```python
from build123d import *

# Parameters (mm, degrees)
SKETCH1_W           = 120.675
SKETCH1_H           = 1.5875
SKETCH6_R           = 7.9375
BOSS_EXTRUDE1_DEPTH = 101.6
SKETCH7_R           = 23.308025585
CUT_EXTRUDE3_DEPTH  = 19.075
SKETCH4_R           = 12.7
CUT_EXTRUDE4_DEPTH  = 41.50106


with BuildPart() as part:
    # Sketch1 → Revolve1 (revolve)
    with BuildSketch(Plane(origin=(0, 0, 0), x_dir=(1, 0, 0), z_dir=(0, 1, 0))):
        with Locations((79.5875, 8.73125)):
            Rectangle(SKETCH1_W, SKETCH1_H)
    revolve(axis=Axis((157.324, 0, 0), (-1, 0, 0)))

    # Sketch6 → Boss-Extrude1 (add)
    with BuildSketch(Plane.ZY.offset(-19.25)):
        with Locations(Location((0, 0, 0), (0, 0, 180))):
            Circle(SKETCH6_R)
    extrude(amount=-BOSS_EXTRUDE1_DEPTH)

    # Sketch7 → Cut-Extrude3 (cut)
    with BuildSketch(Plane(origin=(120.85, 0, 0), x_dir=(0, 0, -1), z_dir=(1, 0, 0))):
        Circle(SKETCH7_R)
    extrude(amount=CUT_EXTRUDE3_DEPTH, mode=Mode.SUBTRACT)

    # Sketch4 → Cut-Extrude4 (cut)
    with BuildSketch(Plane(origin=(0, 0, 0), x_dir=(0, 0, -1), z_dir=(1, 0, 0))):
        Circle(SKETCH4_R)
        Polygon((-9.235721046, 0.808020891), (-8.681700155, 0.254), (-8.681700155, -0.254), (-9.235721046, -0.808020891), (-8.593912259, -1.257420242), (-8.505698985, -1.75770258), (-8.955098336, -2.399511367), (-8.245002688, -2.730634406), (-8.071256455, -3.207998257), (-8.402379494, -3.918093905), (-7.645572882, -4.120879625), (-7.391572882, -4.56082053), (-7.594358603, -5.317627141), (-6.813836213, -5.385914002), (-6.487300108, -5.775064579), (-6.555586968, -6.555586968), (-5.775064579, -6.487300108), (-5.385914002, -6.813836213), (-5.317627141, -7.594358603), (-4.56082053, -7.391572882), (-4.120879625, -7.645572882), (-3.918093905, -8.402379494), (-3.207998257, -8.071256455), (-2.730634406, -8.245002688), (-2.399511367, -8.955098336), (-1.75770258, -8.505698985), (-1.257420242, -8.593912259), (-0.808020891, -9.235721046), (-0.254, -8.681700155), (0.254, -8.681700155), (0.808020891, -9.235721046), (1.257420242, -8.593912259), (1.75770258, -8.505698985), (2.399511367, -8.955098336), (2.730634406, -8.245002688), (3.207998257, -8.071256455), (3.918093905, -8.402379494), (4.120879625, -7.645572882), (4.56082053, -7.391572882), (5.317627141, -7.594358603), (5.385914002, -6.813836213), (5.775064579, -6.487300108), (6.555586968, -6.555586968), (6.487300108, -5.775064579), (6.813836213, -5.385914002), (7.594358603, -5.317627141), (7.391572882, -4.56082053), (7.645572882, -4.120879625), (8.402379494, -3.918093905), (8.071256455, -3.207998257), (8.245002688, -2.730634406), (8.955098336, -2.399511367), (8.505698985, -1.75770258), (8.593912259, -1.257420242), (9.235721046, -0.808020891), (8.681700155, -0.254), (8.681700155, 0.254), (9.235721046, 0.808020891), (8.593912259, 1.257420242), (8.505698985, 1.75770258), (8.955098336, 2.399511367), (8.245002688, 2.730634406), (8.071256455, 3.207998257), (8.402379494, 3.918093905), (7.645572882, 4.120879625), (7.391572882, 4.56082053), (7.594358603, 5.317627141), (6.813836213, 5.385914002), (6.487300108, 5.775064579), (6.555586968, 6.555586968), (5.775064579, 6.487300108), (5.385914002, 6.813836213), (5.317627141, 7.594358603), (4.56082053, 7.391572882), (4.120879625, 7.645572882), (3.918093905, 8.402379494), (3.207998257, 8.071256455), (2.730634406, 8.245002688), (2.399511367, 8.955098336), (1.75770258, 8.505698985), (1.257420242, 8.593912259), (0.808020891, 9.235721046), (0.254, 8.681700155), (-0.254, 8.681700155), (-0.808020891, 9.235721046), (-1.257420242, 8.593912259), (-1.75770258, 8.505698985), (-2.399511367, 8.955098336), (-2.730634406, 8.245002688), (-3.207998257, 8.071256455), (-3.918093905, 8.402379494), (-4.120879625, 7.645572882), (-4.56082053, 7.391572882), (-5.317627141, 7.594358603), (-5.385914002, 6.813836213), (-5.775064579, 6.487300108), (-6.555586968, 6.555586968), (-6.487300108, 5.775064579), (-6.813836213, 5.385914002), (-7.594358603, 5.317627141), (-7.391572882, 4.56082053), (-7.645572882, 4.120879625), (-8.402379494, 3.918093905), (-8.071256455, 3.207998257), (-8.245002688, 2.730634406), (-8.955098336, 2.399511367), (-8.505698985, 1.75770258), (-8.593912259, 1.257420242), align=None, mode=Mode.SUBTRACT)
    extrude(amount=CUT_EXTRUDE4_DEPTH, mode=Mode.SUBTRACT)


solid = part.part
```
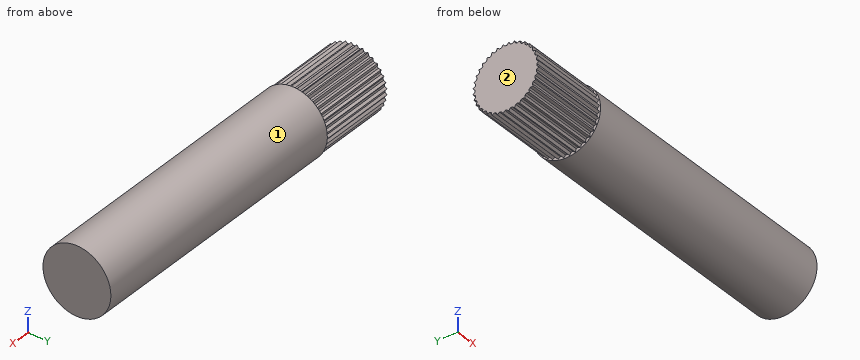
Here's how the part is built. I have some questions about the finished solid (model axes, mm). Face numbers are marked on the shaded views. Round coordinates to 2 decimals unless told otherwise and drop trailing zeros. Order: outer loops, then holes, each group sorted by start corner. A loop starts at its lowest first (then second) coordinate and runs counter-clockwise, first axis right, second up. Notation, with made-up numbers: (-12.5, -22) -> (19.5, -22) arc R7 ccw to (19.5, -10) -> close; hole circle Ø6 at (10.5, 70.25). An arc over 180 degrees is marked (long way). Use a Markdown table: item, result. Add a question column.
(1) Suppose I cut it at A-A, the plane x = 68. Please give me the cut outline in (y, z) (3 decimals), and give its area (3 significant figures).
(2) If we mould it in two halves opening along Z, with no side actions, what happens to the marked faces 1 and 2? For each: released by +Z, released by -Z, zero draft, split by the parting line, or undercut.
(3) I need wall thicknesses on line 1 along Z through (x, y) = (53.5, 2.25); line 2 along Y through (x, z) = (25, -2.75); line 3 along Y through (x, z) = (111, 6). Which ranges of each line are inside material? Lowest first, please.
(4) For pin 1 Ø0.6 at (x, z) = (32.5, 0) entering from +Y; pin 2 Ø8 at (x, z) = (44.5, -6.5) entering from +Y; pin 3 Ø3 at (x, y) = (45.5, 6) entering from -Z (3 decimals), each with a flat end and sliding along its axis, tell me the tip position at first contact or that it passes through.
Verdict:
| question | item | result |
|---|---|---|
| 1 | outline | circle Ø19.05 at (0, 0) |
| 1 | area | 285 mm2 |
| 2 | face 1 | split by the parting line |
| 2 | face 2 | zero draft |
| 3 | line 1 | -9.26 to 9.26 |
| 3 | line 2 | -8.24 to 8.24 |
| 3 | line 3 | -7.4 to 7.4 |
| 4 | pin 1 | y = 8.73 |
| 4 | pin 2 | y = 9.19 |
| 4 | pin 3 | z = -8.395 |
